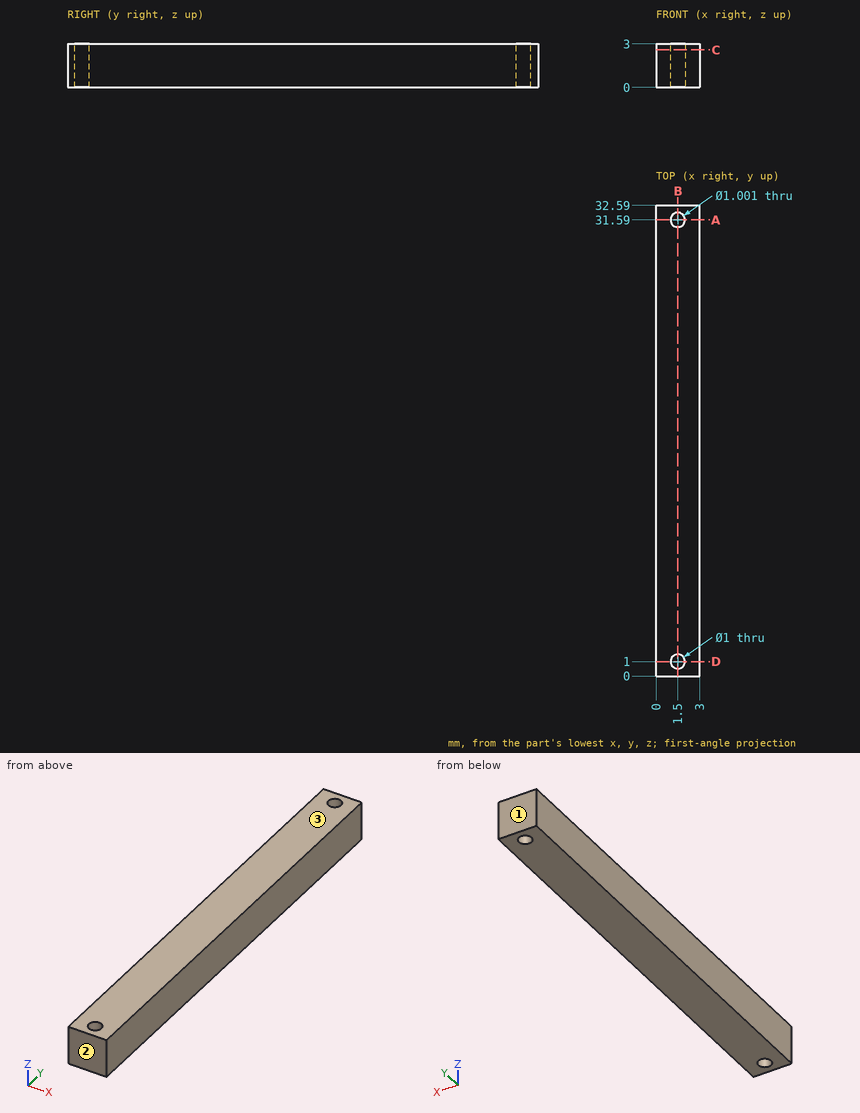
For this review, use the dimensioned drawing (mm, ordinates from the lowest corner) and the shaded views. Coordinates: 2 decimals unless noted, no trailing zeros. Loops run counter-clockwise (first coordinate to the right, second up) from the corner with the lowest first, then second, coordinate; pieces in that order, holes last. Notation, with made-up numbers: (-13, -29) -> (29, -29) arc R16 cw to (29, -8) -> close; hole circle Ø3 at (48, 54). An arc over 180 degrees is marked (long way). Return JSON: item names as keys, results as strings. Group by question number.
(1) Consider section C-C, the plane z = 2.6. Give the boundary of the cut face in (x, y).
(2) Mouldability with a two-part tool opening along Y and no side actions: class the marked faces 1, 2 and 3 as pulls with the +Y half, pulls with the -Y half, needs draft (parallel to the pull), parting line crosses it, or undercut.
(3) To check wall thickness, follow L1, parallel to Y at x = 1.5, z = 1.7; L2, parallel to Y at x = 1.2, z = 0.8. State the ranges of each line that lie inside material, in increasing order.
(4) Consider section B-B, the plane x = 1.5. Give the boundary of the cut face in (y, z).
(5) Consider section A-A, the plane y = 31.59. Give the boundary of the cut face in (x, z).
(6) For pin 1 Ø0.6 at (x, y) = (1.5, 31.59) entering from +Z, flat-tipped, find the tip position at first contact; note if it passes through.
Results below:
{
 "1": {"outline": "(0, 0) -> (3, 0) -> (3, 32.59) -> (0, 32.59) -> close; hole circle Ø1 at (1.5, 1); hole circle Ø1 at (1.5, 31.59)"},
 "2": {"face 1": "pulls with the +Y half", "face 2": "pulls with the -Y half", "face 3": "needs draft"},
 "3": {"L1": "y = 0 to 0.5, 1.5 to 31.09, 32.09 to 32.59", "L2": "y = 0 to 0.6, 1.4 to 31.19, 31.99 to 32.59"},
 "4": {"outline": "(0, 0) -> (0.5, 0) -> (0.5, 3) -> (0, 3) -> close; (1.5, 0) -> (31.09, 0) -> (31.09, 3) -> (1.5, 3) -> close; (32.09, 0) -> (32.59, 0) -> (32.59, 3) -> (32.09, 3) -> close"},
 "5": {"outline": "(0, 0) -> (1, 0) -> (1, 3) -> (0, 3) -> close; (2, 0) -> (3, 0) -> (3, 3) -> (2, 3) -> close"},
 "6": {"pin 1": "passes through"}
}
